Could you check a few things on this model? Use its own coordinates, in mm. Face numbers are marked on the shaded views. A direction names the side the tool comes from. Round coordinates to 2 decimals unless told otherwise and drop trailing zeros. Write each loop counter-clockwise with the first axis right and the second up, starting at its lowest first coordinate (ties: lowest second). Pieces come first, ordered by that corner, then holes. Notation, with made-up numbers: (21.5, 66) -> (76.5, 66) arc R29 cw to (76.5, 95) -> close; hole circle Ø9 at (-25, -17.75). An arc over 180 degrees is marked (long way). Answer in a Markdown table with one row per item. Add a question column.
```python
from build123d import *

# Parameters (mm, degrees)
BOSS_EXTRUDE1_DEPTH              = 19.05
F_21_64_0_32813_DIAMETER_HOLE1_D = 8.334502


with BuildPart() as part:
    # Sketch2 → Boss-Extrude1 (new body)
    with BuildSketch(Plane.XY):
        Polygon((0, 0), (12.7, 0), (12.7, -40.64), (63.5, -44.7675), (113.03, -40.64), (113.03, -32.0675), (109.22, -32.0675), (109.22, -35.56), (63.5, -39.37), (19.05, -35.56), (19.05, 0), (19.05, 82.55), (0, 82.55), align=None)
        Polygon((-12.7, 0), (0, 0), (0, 82.55), (-19.05, 82.55), (-19.05, 0), (-19.05, -35.56), (-63.5, -39.37), (-109.22, -35.56), (-109.22, -32.0675), (-113.03, -32.0675), (-113.03, -40.64), (-63.5, -44.7675), (-12.7, -40.64), align=None)
    extrude(amount=BOSS_EXTRUDE1_DEPTH)

    # 21/64 (0.32813) Diameter Hole1 (through all)
    with Locations(Plane.XY.offset(19.05)):
        with Locations((0, 25.4), (0, 63.5)):
            Hole(F_21_64_0_32813_DIAMETER_HOLE1_D / 2)


solid = part.part
```
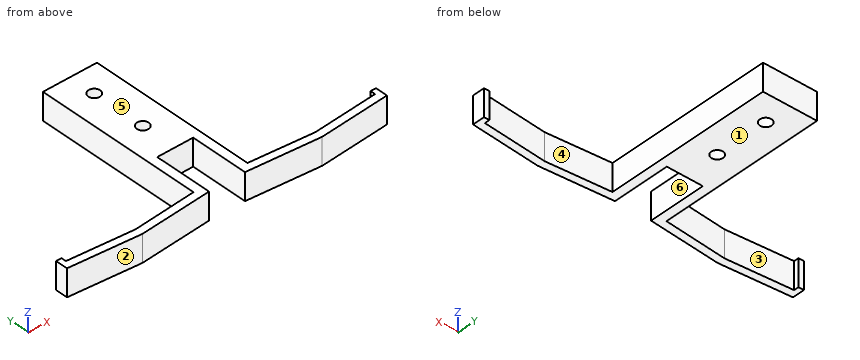
(1) On a 3-axis mill with a long thin cutter (end or side, diameter ignored), from which of +Z, -Z, +X, -X, +Y, -Y can I reach the whole of each face in a straight line? I mean the marked faces 4, 5 and 6. Say none if no direction works.
(2) Suppose I cut it at B-B, the plane y = 25.4. Please give me the cut outline in (x, z).
(3) Suppose I cut it at A-A, the plane x = 0. Please give me the cut outline in (y, z), then the cut area to 3 significant figures.
(4) Suppose I cut it at D-D, the plane y = -5. Please give me the cut outline in (x, z), then the cut area to 3 significant figures.
(5) For P1, Ø3, axis at x = -111.5, z = 12.5, coming from the +Y side; P2, Ø4, axis at y = -2.5, z = 2.5, coming from the +X side; P3, Ø5.5, axis at y = 51.5, z = 8.5, coming from the -X side; P4, Ø5, axis at x = 0, y = 25.4, coming from the -Z side, each with a flat end and sliding along its axis, tell me the tip position at first contact or that it passes through.
(6) I need wall thicknesses on L1, parallel to Y at x = 0, z = 8.5; L2, parallel to X at y = -21.5, z = 2.75; L3, parallel to X at y = 54, z = 5. Which ranges of each line are inside material? Lowest first, please.
(7) If we mould it in two halves opening along X, with no side actions, what happens to the marked faces 1, 2 and 3? For each: pulls with the +X half, pulls with the -X half, needs draft (parallel to the pull), parting line crosses it, or undercut.
(8) Suppose I cut it at C-C, the plane z = 16.25. Please give me the cut outline in (x, y), then the cut area to 3 significant figures.
Response:
| question | item | result |
|---|---|---|
| 1 | face 4 | +Z, -Z, +Y |
| 1 | face 5 | +Z, +X, -X, +Y, -Y |
| 1 | face 6 | +Z, -Z, -Y |
| 2 | outline | (-19.05, 0) -> (-4.17, 0) -> (-4.17, 19.05) -> (-19.05, 19.05) -> close; (4.17, 0) -> (19.05, 0) -> (19.05, 19.05) -> (4.17, 19.05) -> close |
| 3 | outline | (0, 0) -> (21.23, 0) -> (21.23, 19.05) -> (0, 19.05) -> close; (29.57, 0) -> (59.33, 0) -> (59.33, 19.05) -> (29.57, 19.05) -> close; (67.67, 0) -> (82.55, 0) -> (82.55, 19.05) -> (67.67, 19.05) -> close |
| 3 | area | 1,260 mm² |
| 4 | outline | (-19.05, 0) -> (-12.7, 0) -> (-12.7, 19.05) -> (-19.05, 19.05) -> close; (12.7, 0) -> (19.05, 0) -> (19.05, 19.05) -> (12.7, 19.05) -> close |
| 4 | area | 242 mm² |
| 5 | P1 | y = -32.07 |
| 5 | P2 | x = 19.05 |
| 5 | P3 | x = -19.05 |
| 5 | P4 | through |
| 6 | L1 | 0 to 21.23, 29.57 to 59.33, 67.67 to 82.55 |
| 6 | L2 | -19.05 to -12.7, 12.7 to 19.05 |
| 6 | L3 | -19.05 to 19.05 |
| 7 | face 1 | needs draft |
| 7 | face 2 | pulls with the -X half |
| 7 | face 3 | undercut |
| 8 | outline | (-113.03, -40.64) -> (-63.5, -44.77) -> (-12.7, -40.64) -> (-12.7, 0) -> (12.7, 0) -> (12.7, -40.64) -> (63.5, -44.77) -> (113.03, -40.64) -> (113.03, -32.07) -> (109.22, -32.07) -> (109.22, -35.56) -> (63.5, -39.37) -> (19.05, -35.56) -> (19.05, 82.55) -> (-19.05, 82.55) -> (-19.05, -35.56) -> (-63.5, -39.37) -> (-109.22, -35.56) -> (-109.22, -32.07) -> (-113.03, -32.07) -> close; hole circle Ø8.33 at (0, 25.4); hole circle Ø8.33 at (0, 63.5) |
| 8 | area | 4,600 mm² |
